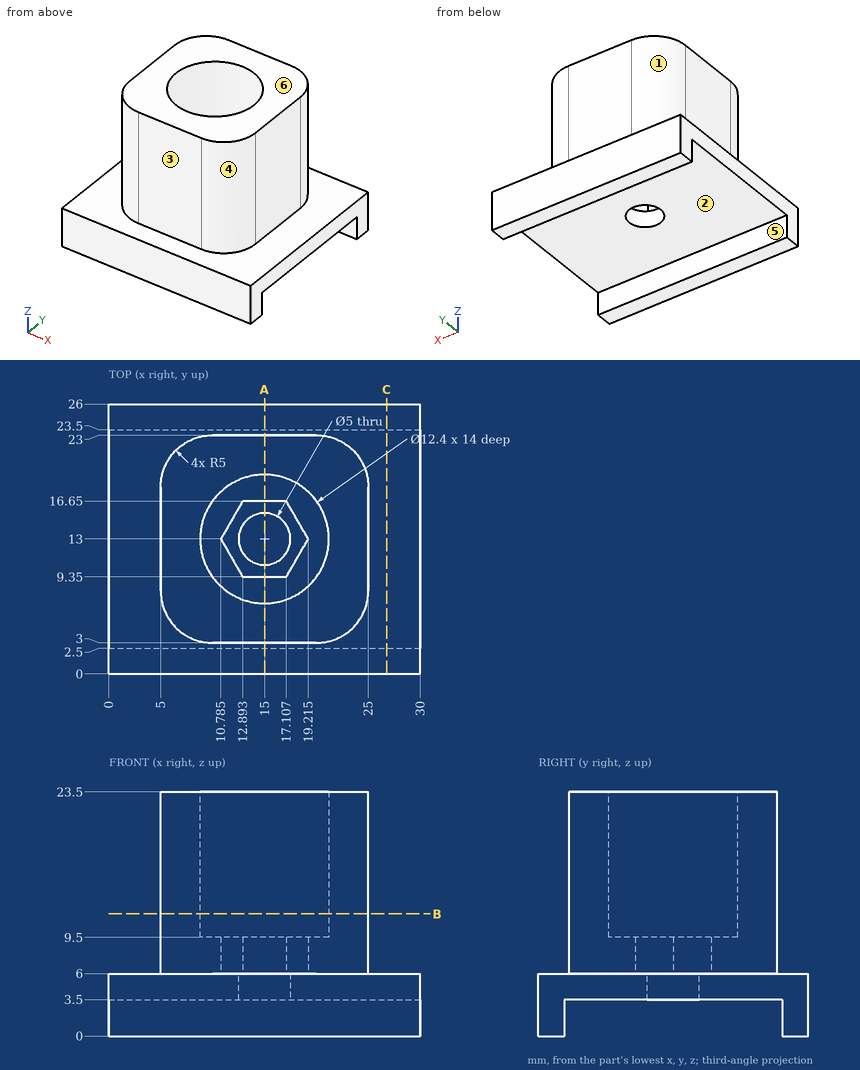
Check sheet for the drawn part. Datum: minimum x, y, z corner. Units: mm. A direction names the side the tool comes from. Round coordinates to 2 decimals unless told otherwise and drop trailing zeros. Write each loop counter-clockwise with the first axis right and the second up, starting at its lowest first coordinate (ties: lowest second). Pieces come first, ordered by that corner, then holes. Notation, with made-up numbers: (3, 58) -> (32, 58) arc R3 cw to (32, 62) -> close; hole circle Ø4 at (-31.5, 9). An arc over 180 degrees is marked (long way). Put each result on its own line as item: value.
(1) Sectioned sample at A-A (x = 15). Enter the section's corners in (y, z), plus the area to 3 significant figures.
Values found:
outline: (0, 0) -> (2.5, 0) -> (2.5, 3.5) -> (10.5, 3.5) -> (10.5, 6) -> (9.35, 6) -> (9.35, 9.5) -> (6.8, 9.5) -> (6.8, 23.5) -> (3, 23.5) -> (3, 6) -> (0, 6) -> close; (15.5, 3.5) -> (23.5, 3.5) -> (23.5, 0) -> (26, 0) -> (26, 6) -> (23, 6) -> (23, 23.5) -> (19.2, 23.5) -> (19.2, 9.5) -> (16.65, 9.5) -> (16.65, 6) -> (15.5, 6) -> close
area: 221 mm^2
(2) Go/stop test with flat-tipped pins: pin 1 Ø1 at (y, z) = (15.5, 15.5) entering from -X; pin 2 Ø6.5 at (x, y) = (15, 13) entering from +Z; pin 3 Ø4 at (x, z) = (22, 2) entering from -Y; pin 4 Ø6 at (x, y) = (16, 11.5) entering from +Z. Record where each tip stops, or that it passes through.
Values found:
pin 1: stops at x = 5
pin 2: stops at z = 6
pin 3: stops at y = 0
pin 4: stops at z = 9.5
(3) Mould release check, pull along Y, two halves, no side actions. Record for the marked faces 4, 5 and 6: released by +Y, released by -Y, zero draft, split by the parting line, or undercut.
Values found:
face 4: released by -Y
face 5: undercut
face 6: zero draft
(4) Material ranges on line 1 (Y direction, x = 15, z = 4.35); line 2 (Y direction, x = 16, z = 3); line 3 (Z direction, x = 16.25, y = 7.5), recorded low to high.
Values found:
line 1: y = 0 to 10.5, 15.5 to 26
line 2: y = 0 to 2.5, 23.5 to 26
line 3: z = 3.5 to 9.5
(5) Sectioned sample at C-C (x = 26.75). Enter the section's corners in (y, z).
Values found:
outline: (0, 0) -> (2.5, 0) -> (2.5, 3.5) -> (23.5, 3.5) -> (23.5, 0) -> (26, 0) -> (26, 6) -> (0, 6) -> close
(6) Tool access check on the marked faces 1, 2 and 3. Record the directions out of +Z, -Z, +X, -X, +Y, -Y that give a thin tool (end or side, any length) a straight path to the whole face; none if there is none.
Values found:
face 1: +Z, -X, +Y
face 2: -Z, +X, -X
face 3: +Z, +X, -X, -Y
(7) Sectioned sample at B-B (z = 11.75). Enter the section's corners in (x, y).
Values found:
outline: (5, 8) arc R5 ccw to (10, 3) -> (20, 3) arc R5 ccw to (25, 8) -> (25, 18) arc R5 ccw to (20, 23) -> (10, 23) arc R5 ccw to (5, 18) -> close; hole circle Ø12.4 at (15, 13)
